Geometry check sheet. Reference: the model listing, model coordinates, mm. Give positions to 0.01 mm unless a question says otherwise; leave off trailing zeros. Order: outer loops, then holes, each group sorted by start corner. A loop starts at its lowest first (then second) coordinate and runs counter-clockwise, first axis right, second up. Notation, with made-up numbers: M 72,50 L 86,50 A26 ccw 86,73 Z; hole C 69.5,-16 d7. An arc over 180 degrees is marked long. Answer as CSV lines item,"result". Start each with the question number.
Q1. Section check D-D, the plane z = 0.3. Count the separate pieces of the cut face and the enclosed holes in it, then the cut area to 3 significant figures.
Q2. Thickness scan on line 1 (Y direction, x = 13.93, z = 0.45); line 2 (X direction, y = 19, z = 0.75); line 3 (Y direction, x = 21.5, z = 0.4). Record the ranges inside material, lowest first.
Q3. Mould release check, pull along X, two halves, no side actions. Record for faces 1 (the cylindrical face through (10.31, 4.62, 0.79)), 2 (the cylindrical face through (16.409, 20.167, 0.789)), 3 (the flat face through (0, 12, 1)), 4 (the flat face through (12, 12, 1.6)): +X half, -X half, draft (parallel to the pull), parting line (faces both ways), or undercut.
Q4. Section check B-B, the plane y = 19. Record the boundary of the cut face in (x, z), then the cut area to 3 significant figures.
Q5. Section check C-C, the plane x = 21.5. Record the boundary of the cut face in (y, z), then the cut area to 3 significant figures.
Q6. Section check A-A, the plane x = 12. Record the boundary of the cut face in (y, z).
Autodesk Inventor part; units mm, degrees
ref_plane "YZ Plane" through (0, 0, 0) normal (1, 0, 0) x (0, 1, 0)
ref_plane "XZ Plane" through (0, 0, 0) normal (0, 1, 0) x (-1, 0, 0)
ref_plane "XY Plane" through (0, 0, 0) normal (0, 0, 1) x (1, 0, 0)
sketch "Sketch1" plane through (0, 0, 0) normal (0, 0, 1) x (1, 0, 0)
  line L0 (0, -0.5) -> (24, -0.5)
  line L1 (24, -0.5) -> (24, 24.5)
  line L2 (24, 24.5) -> (0, 24.5)
  line L3 (0, 24.5) -> (0, -0.5)
  circle A0 centre (13.93, 20.61) radius 0.45
  circle A1 centre (17.22, 20.91) radius 1.1
  circle A2 centre (6.75, 20.91) radius 1.1
  circle A3 centre (13.93, 19) radius 0.45
  circle A4 centre (12, 20.61) radius 0.45
  circle A5 centre (12, 19) radius 0.45
  circle A6 centre (10.07, 20.61) radius 0.45
  circle A7 centre (10.07, 19) radius 0.45
  circle A8 centre (10.07, 3.39) radius 0.45
  circle A9 centre (6.78, 3.1) radius 1.1
  circle A10 centre (17.25, 3.1) radius 1.1
  circle A11 centre (10.07, 5) radius 0.45
  circle A12 centre (12, 3.39) radius 0.45
  circle A13 centre (12, 5) radius 0.45
  circle A14 centre (13.93, 3.39) radius 0.45
  circle A15 centre (13.93, 5) radius 0.45
  circle A16 centre (2.5, 21) radius 1.5
  circle A17 centre (21.5, 21) radius 1.5
  circle A18 centre (21.5, 3) radius 1.5
  circle A19 centre (2.5, 3) radius 1.5
extrude "untitled.brd_Outline" add sketch "Sketch1" along normal blind 1.6
properties part number "untitled.brd_Outline"
Answer block:
1,separate pieces,"1"
1,enclosed holes,"20"
1,area,"549 mm2"
2,line 1,"y = -0.5 to 2.94, 3.84 to 4.55, 5.45 to 18.55, 19.45 to 20.16, 21.06 to 24.5"
2,line 2,"x = 0 to 9.62, 10.52 to 11.55, 12.45 to 13.48, 14.38 to 24"
2,line 3,"y = -0.5 to 1.5, 4.5 to 19.5, 22.5 to 24.5"
3,face 1,"undercut"
3,face 2,"undercut"
3,face 3,"-X half"
3,face 4,"draft"
4,outline,"M 0,0 L 9.62,0 L 9.62,1.6 L 0,1.6 Z; M 10.52,0 L 11.55,0 L 11.55,1.6 L 10.52,1.6 Z; M 12.45,0 L 13.48,0 L 13.48,1.6 L 12.45,1.6 Z; M 14.38,0 L 24,0 L 24,1.6 L 14.38,1.6 Z"
4,area,"34.1 mm2"
5,outline,"M -0.5,0 L 1.5,0 L 1.5,1.6 L -0.5,1.6 Z; M 4.5,0 L 19.5,0 L 19.5,1.6 L 4.5,1.6 Z; M 22.5,0 L 24.5,0 L 24.5,1.6 L 22.5,1.6 Z"
5,area,"30.4 mm2"
6,outline,"M -0.5,0 L 2.94,0 L 2.94,1.6 L -0.5,1.6 Z; M 3.84,0 L 4.55,0 L 4.55,1.6 L 3.84,1.6 Z; M 5.45,0 L 18.55,0 L 18.55,1.6 L 5.45,1.6 Z; M 19.45,0 L 20.16,0 L 20.16,1.6 L 19.45,1.6 Z; M 21.06,0 L 24.5,0 L 24.5,1.6 L 21.06,1.6 Z"
